```python
from build123d import *

# Parameters (mm, degrees)
F0_W     = 914.4
F0_H     = 914.4
F0_R     = 1.5875
F0_R_2   = 2.1
F0_R_3   = 3.15
F0_R_4   = 1.65
F0_R_5   = 68
F1_DEPTH = 1.27


with BuildPart() as f1:
    # F0 (on Top) → F1 (new body)
    with BuildSketch(Plane.XY):
        with Locations((-14.713987, 60.998162)):
            Rectangle(F0_W, F0_H)
        with Locations((-465.563987, -389.851838)):
            Circle(F0_R, mode=Mode.SUBTRACT)
        with Locations((-332.213987, -389.851838)):
            Circle(F0_R, mode=Mode.SUBTRACT)
        with Locations((-465.563987, -277.139338)):
            Circle(F0_R, mode=Mode.SUBTRACT)
        with Locations((-429.083987, -222.338838)):
            Circle(F0_R_2, mode=Mode.SUBTRACT)
        Polygon((-238.995987, -66.763838), (-238.995987, -377.151838), (-238.995987, -377.558238), (-425.431987, -377.558238), (-425.431987, -377.151838), (-425.431987, -66.763838), (-425.431987, -66.357438), (-238.995987, -66.357438), align=None, mode=Mode.SUBTRACT)
        with Locations((-198.863987, -389.851838)):
            Circle(F0_R, mode=Mode.SUBTRACT)
        with Locations((-148.063987, -389.851838)):
            Circle(F0_R, mode=Mode.SUBTRACT)
        with Locations((-235.343987, -267.338838)):
            Circle(F0_R_2, mode=Mode.SUBTRACT)
        with Locations((-198.863987, -243.801838)):
            Circle(F0_R_3, mode=Mode.SUBTRACT)
        with Locations((-235.343987, -222.338838)):
            Circle(F0_R_2, mode=Mode.SUBTRACT)
        with Locations((-111.583987, -267.338838)):
            Circle(F0_R_2, mode=Mode.SUBTRACT)
        with Locations((-111.583987, -222.338838)):
            Circle(F0_R_2, mode=Mode.SUBTRACT)
        Polygon((-107.931987, -66.763838), (-107.931987, -66.357438), (78.504013, -66.357438), (78.504013, -66.763838), (78.504013, -377.151838), (78.504013, -377.558238), (-107.931987, -377.558238), (-107.931987, -377.151838), align=None, mode=Mode.SUBTRACT)
        with Locations((-465.563987, -164.426838)):
            Circle(F0_R, mode=Mode.SUBTRACT)
        with Locations((-429.083987, -127.338838)):
            Circle(F0_R_2, mode=Mode.SUBTRACT)
        with Locations((-465.563987, -51.714338)):
            Circle(F0_R, mode=Mode.SUBTRACT)
        with Locations((-465.563987, 60.998162)):
            Circle(F0_R, mode=Mode.SUBTRACT)
        with Locations((-384.713987, 8.498162)):
            Circle(F0_R_4, mode=Mode.SUBTRACT)
        with Locations((-279.713987, 8.498162)):
            Circle(F0_R_4, mode=Mode.SUBTRACT)
        with Locations((-198.863987, -164.426838)):
            Circle(F0_R, mode=Mode.SUBTRACT)
        with Locations((-148.063987, -164.426838)):
            Circle(F0_R, mode=Mode.SUBTRACT)
        with Locations((-198.863987, 60.998162)):
            Circle(F0_R, mode=Mode.SUBTRACT)
        with Locations((-148.063987, 60.998162)):
            Circle(F0_R, mode=Mode.SUBTRACT)
        with Locations((-67.213987, 8.498162)):
            Circle(F0_R_4, mode=Mode.SUBTRACT)
        with Locations((-14.713987, -389.851838)):
            Circle(F0_R, mode=Mode.SUBTRACT)
        with Locations((118.636013, -389.851838)):
            Circle(F0_R, mode=Mode.SUBTRACT)
        with Locations((169.436013, -389.851838)):
            Circle(F0_R, mode=Mode.SUBTRACT)
        with Locations((82.156013, -222.338838)):
            Circle(F0_R_2, mode=Mode.SUBTRACT)
        with Locations((205.916013, -267.338838)):
            Circle(F0_R_2, mode=Mode.SUBTRACT)
        with Locations((169.436013, -243.801838)):
            Circle(F0_R_3, mode=Mode.SUBTRACT)
        with Locations((205.916013, -222.338838)):
            Circle(F0_R_2, mode=Mode.SUBTRACT)
        with Locations((302.786013, -389.851838)):
            Circle(F0_R, mode=Mode.SUBTRACT)
        with Locations((436.136013, -389.851838)):
            Circle(F0_R, mode=Mode.SUBTRACT)
        Polygon((209.568013, -377.558238), (209.568013, -377.151838), (209.568013, -66.763838), (209.568013, -66.357438), (396.004013, -66.357438), (396.004013, -66.763838), (396.004013, -377.151838), (396.004013, -377.558238), align=None, mode=Mode.SUBTRACT)
        with Locations((436.136013, -277.139338)):
            Circle(F0_R, mode=Mode.SUBTRACT)
        with Locations((399.656013, -222.338838)):
            Circle(F0_R_2, mode=Mode.SUBTRACT)
        with Locations((82.156013, -127.338838)):
            Circle(F0_R_2, mode=Mode.SUBTRACT)
        with Locations((118.636013, -164.426838)):
            Circle(F0_R, mode=Mode.SUBTRACT)
        with Locations((169.436013, -164.426838)):
            Circle(F0_R, mode=Mode.SUBTRACT)
        with Locations((37.786013, 8.498162)):
            Circle(F0_R_4, mode=Mode.SUBTRACT)
        with Locations((436.136013, -164.426838)):
            Circle(F0_R, mode=Mode.SUBTRACT)
        with Locations((399.656013, -127.338838)):
            Circle(F0_R_2, mode=Mode.SUBTRACT)
        with Locations((250.286013, 8.498162)):
            Circle(F0_R_4, mode=Mode.SUBTRACT)
        with Locations((436.136013, -51.714338)):
            Circle(F0_R, mode=Mode.SUBTRACT)
        with Locations((355.286013, 8.498162)):
            Circle(F0_R_4, mode=Mode.SUBTRACT)
        with Locations((-384.713987, 113.498162)):
            Circle(F0_R_4, mode=Mode.SUBTRACT)
        with Locations((-465.563987, 173.710662)):
            Circle(F0_R, mode=Mode.SUBTRACT)
        with Locations((-332.213987, 60.998162)):
            Circle(F0_R_5, mode=Mode.SUBTRACT)
        with Locations((-279.713987, 113.498162)):
            Circle(F0_R_4, mode=Mode.SUBTRACT)
        with Locations((-429.083987, 249.335162)):
            Circle(F0_R_2, mode=Mode.SUBTRACT)
        with Locations((-465.563987, 286.423162)):
            Circle(F0_R, mode=Mode.SUBTRACT)
        with Locations((-14.713987, 60.998162)):
            Circle(F0_R_5, mode=Mode.SUBTRACT)
        with Locations((-67.213987, 113.498162)):
            Circle(F0_R_4, mode=Mode.SUBTRACT)
        with Locations((-198.863987, 286.423162)):
            Circle(F0_R, mode=Mode.SUBTRACT)
        with Locations((-148.063987, 286.423162)):
            Circle(F0_R, mode=Mode.SUBTRACT)
        with Locations((-429.083987, 344.335162)):
            Circle(F0_R_2, mode=Mode.SUBTRACT)
        with Locations((-465.563987, 399.135662)):
            Circle(F0_R, mode=Mode.SUBTRACT)
        Polygon((-238.995987, 499.554562), (-238.995987, 499.148162), (-238.995987, 188.760162), (-238.995987, 188.353762), (-425.431987, 188.353762), (-425.431987, 188.760162), (-425.431987, 499.148162), (-425.431987, 499.554562), align=None, mode=Mode.SUBTRACT)
        with Locations((-465.563987, 511.848162)):
            Circle(F0_R, mode=Mode.SUBTRACT)
        with Locations((-332.213987, 511.848162)):
            Circle(F0_R, mode=Mode.SUBTRACT)
        with Locations((-235.343987, 344.335162)):
            Circle(F0_R_2, mode=Mode.SUBTRACT)
        with Locations((-198.863987, 365.798162)):
            Circle(F0_R_3, mode=Mode.SUBTRACT)
        with Locations((-235.343987, 389.335162)):
            Circle(F0_R_2, mode=Mode.SUBTRACT)
        with Locations((-111.583987, 344.335162)):
            Circle(F0_R_2, mode=Mode.SUBTRACT)
        Polygon((78.504013, 499.554562), (78.504013, 499.148162), (78.504013, 188.760162), (78.504013, 188.353762), (-107.931987, 188.353762), (-107.931987, 188.760162), (-107.931987, 499.148162), (-107.931987, 499.554562), align=None, mode=Mode.SUBTRACT)
        with Locations((-111.583987, 389.335162)):
            Circle(F0_R_2, mode=Mode.SUBTRACT)
        with Locations((-198.863987, 511.848162)):
            Circle(F0_R, mode=Mode.SUBTRACT)
        with Locations((-148.063987, 511.848162)):
            Circle(F0_R, mode=Mode.SUBTRACT)
        with Locations((37.786013, 113.498162)):
            Circle(F0_R_4, mode=Mode.SUBTRACT)
        with Locations((118.636013, 60.998162)):
            Circle(F0_R, mode=Mode.SUBTRACT)
        with Locations((169.436013, 60.998162)):
            Circle(F0_R, mode=Mode.SUBTRACT)
        with Locations((82.156013, 249.335162)):
            Circle(F0_R_2, mode=Mode.SUBTRACT)
        with Locations((118.636013, 286.423162)):
            Circle(F0_R, mode=Mode.SUBTRACT)
        with Locations((169.436013, 286.423162)):
            Circle(F0_R, mode=Mode.SUBTRACT)
        with Locations((250.286013, 113.498162)):
            Circle(F0_R_4, mode=Mode.SUBTRACT)
        with Locations((302.786013, 60.998162)):
            Circle(F0_R_5, mode=Mode.SUBTRACT)
        with Locations((355.286013, 113.498162)):
            Circle(F0_R_4, mode=Mode.SUBTRACT)
        with Locations((436.136013, 60.998162)):
            Circle(F0_R, mode=Mode.SUBTRACT)
        with Locations((436.136013, 173.710662)):
            Circle(F0_R, mode=Mode.SUBTRACT)
        with Locations((399.656013, 249.335162)):
            Circle(F0_R_2, mode=Mode.SUBTRACT)
        with Locations((436.136013, 286.423162)):
            Circle(F0_R, mode=Mode.SUBTRACT)
        with Locations((82.156013, 344.335162)):
            Circle(F0_R_2, mode=Mode.SUBTRACT)
        with Locations((205.916013, 344.335162)):
            Circle(F0_R_2, mode=Mode.SUBTRACT)
        with Locations((169.436013, 365.798162)):
            Circle(F0_R_3, mode=Mode.SUBTRACT)
        with Locations((205.916013, 389.335162)):
            Circle(F0_R_2, mode=Mode.SUBTRACT)
        with Locations((-14.713987, 511.848162)):
            Circle(F0_R, mode=Mode.SUBTRACT)
        with Locations((118.636013, 511.848162)):
            Circle(F0_R, mode=Mode.SUBTRACT)
        with Locations((169.436013, 511.848162)):
            Circle(F0_R, mode=Mode.SUBTRACT)
        Polygon((209.568013, 188.760162), (209.568013, 499.148162), (209.568013, 499.554562), (396.004013, 499.554562), (396.004013, 499.148162), (396.004013, 188.760162), (396.004013, 188.353762), (209.568013, 188.353762), align=None, mode=Mode.SUBTRACT)
        with Locations((399.656013, 344.335162)):
            Circle(F0_R_2, mode=Mode.SUBTRACT)
        with Locations((436.136013, 399.135662)):
            Circle(F0_R, mode=Mode.SUBTRACT)
        with Locations((302.786013, 511.848162)):
            Circle(F0_R, mode=Mode.SUBTRACT)
        with Locations((436.136013, 511.848162)):
            Circle(F0_R, mode=Mode.SUBTRACT)
    extrude(amount=F1_DEPTH)


solid = f1.part
```
Geometry check sheet. Reference: the model listing, model coordinates, mm. Give positions to 0.01 mm unless a question says otherwise; leave off trailing zeros. Order: outer loops, then holes, each group sorted by start corner. A loop starts at its lowest first (then second) coordinate and runs counter-clockwise, first axis right, second up.
1. Thickness scan on L1, parallel to X at y = -190, z = 0.6; L2, parallel to Y at x = -244, z = 0.6; L3, parallel to X at y = -246.5, z = 1.1. Record the ranges inside material, lowest first.
2. Release check for a two-part mould opening along Y. For faces 1 (the face through (-23.57, 128.42, 0.63)), 2 (the face through (-123, 67, 0)) record: pulls with the +Y half, pulls with the -Y half, needs draft (parallel to the pull), parting line crosses it, or undercut.
3. Section check C-C, the plane z = 0.75. Give the number of separate pieces and of enclosed holes in the cut face, and give its area (3 significant figures).
4. Section check B-B, the plane x = -296. Enter the section's corners in (y, z).
5. Section check A-A, the plane y = 428.5. Enter the section's corners in (x, z), and give its area (3 significant figures).
Values follow:
1. L1: x = -471.91 to -425.43, -239 to -107.93, 78.5 to 209.57, 396 to 442.49
1. L2: y = -396.2 to -377.56, -66.36 to 188.35, 499.55 to 518.2
1. L3: x = -471.91 to -425.43, -239 to -200.49, -197.24 to -107.93, 78.5 to 167.81, 171.06 to 209.57, 396 to 442.49
2. face 1: undercut
2. face 2: needs draft
3. separate pieces: 1
3. enclosed holes: 93
3. area: 444,000 mm2
4. outline: (-396.2, 0) - (-377.56, 0) - (-377.56, 1.27) - (-396.2, 1.27) - close; (-66.36, 0) - (3.44, 0) - (3.44, 1.27) - (-66.36, 1.27) - close; (118.55, 0) - (188.35, 0) - (188.35, 1.27) - (118.55, 1.27) - close; (499.55, 0) - (518.2, 0) - (518.2, 1.27) - (499.55, 1.27) - close
5. outline: (-471.91, 0) - (-425.43, 0) - (-425.43, 1.27) - (-471.91, 1.27) - close; (-239, 0) - (-107.93, 0) - (-107.93, 1.27) - (-239, 1.27) - close; (78.5, 0) - (209.57, 0) - (209.57, 1.27) - (78.5, 1.27) - close; (396, 0) - (442.49, 0) - (442.49, 1.27) - (396, 1.27) - close
5. area: 451 mm2
